Read the model definition and answer for the solid it produces. Units are mm, in the model's axes. Face numbers are marked on the shaded views. A direction names the side the tool comes from. Coordinates: 2 decimals unless noted, no trailing zeros. Order: outer loops, then holes, each group sorted by start corner. A loop starts at its lowest first (then second) coordinate and runs counter-clockwise, first axis right, second up. Notation, with made-up numbers: (-28.5, 16) -> (-15.5, 16) arc R34 cw to (-15.5, 49) -> close; hole circle Ø4 at (83.25, 79). An arc over 180 degrees is marked (long way). Use CSV: the item, a comma, the result in double quotes.
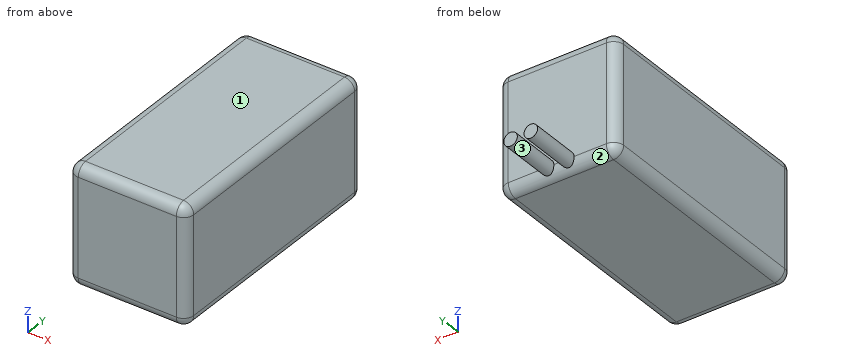
Autodesk Inventor part; units mm, degrees
ref_plane "YZ Plane" through (0, 0, 0) normal (1, 0, 0) x (0, 1, 0)
ref_plane "XZ Plane" through (0, 0, 0) normal (0, 1, 0) x (-1, 0, 0)
ref_plane "XY Plane" through (0, 0, 0) normal (0, 0, 1) x (1, 0, 0)
sketch "Sketch1" plane through (0, 0, 0) normal (0, 1, 0) x (-1, 0, 0)
  line L0 (17.5, 17.5) -> (-17.5, 17.5)
  line L1 (-17.5, 17.5) -> (-17.5, -17.5)
  line L2 (-17.5, -17.5) -> (17.5, -17.5)
  line L3 (17.5, -17.5) -> (17.5, 17.5)
  line L4 (17.5, 17.5) -> (-17.5, -17.5) construction
  line L5 (-17.5, 17.5) -> (17.5, -17.5) construction
  line L6 (0, -17.5) -> (0, -14.5) construction
  line L7 (0, -14.5) -> (3, -14.5) construction
  circle A0 centre (3, -14.5) radius 2
  circle A1 centre (-3, -14.5) radius 2
  point P0 (0, 0)
  dimension "d0" = 35
  dimension "d1" = 35
  dimension "d5" = 3
  dimension "d6" = 3
  dimension "d7" = 4
extrude "Extrusion1" add sketch "Sketch1" along normal blind 72 contours L3 L2 L1 L0 | A0 | A1
extrude "Extrusion2" add sketch "Sketch1" along normal blind 15 from surface at 72 contours A0 | A1
fillet "Fillet1" radius 3 12 edges at (17.5, 36, 17.5) (17.5, 36, -17.5) (-17.5, 36, 17.5) (-17.5, 36, -17.5) (17.5, 72, 0) (0, 72, 17.5) (0, 72, -17.5) (-17.5, 72, 0) (17.5, 0, 0) (0, 0, 17.5) (-17.5, 0, 0) (0, 0, -17.5)
properties part number "Tattu 14,8V 1550 mAh 100C LiPo-Akku XT60"
Item 1: A tool of negligible diameter and unlimited length cuts with its end or side. For the marked faces 1, 2 and 3, from which of +Z, -Z, +X, -X, +Y, -Y can it reach the whole face along a straight path? Write none if from no direction.
Return value:
face 1,"+Z, +X, -X, +Y, -Y"
face 2,"-Z, +Y"
face 3,"+Y"
Item 2: This flat-tipped pin is pushed along its axis until it touches: P1, Ø1.5, axis at x = 0, z = -2.5, coming from the +Y side. Where does it stop, or does it pass through?
Return value:
P1,"stops at y = 72"
Item 3: Straight lines are drawn through the part: line 1 along Y through (x, z) = (-2.5, -11); line 2 along X through (y, z) = (21.5, 16); line 3 along Y through (x, z) = (-1, 16). For each, find the intervals that lie inside material, in ascending order.
Return value:
line 1,"y = 0 to 72"
line 2,"x = -17.1 to 17.1"
line 3,"y = 0.4 to 71.6"
Item 4: Find section B-B, the plane z = 8. Give the vertices of the cut face in (x, y).
Return value:
outline,"(-17.5, 3) arc R3 ccw to (-14.5, 0) -> (14.5, 0) arc R3 ccw to (17.5, 3) -> (17.5, 69) arc R3 ccw to (14.5, 72) -> (-14.5, 72) arc R3 ccw to (-17.5, 69) -> close"
Item 5: Find section C-C, the plane x = -3. Give the vertices of the cut face in (y, z), then the cut area to 3 significant figures.
Return value:
outline,"(0, -14.5) arc R3 ccw to (3, -17.5) -> (69, -17.5) arc R3 ccw to (71.24, -16.5) -> (87, -16.5) -> (87, -12.5) -> (72, -12.5) -> (72, 14.5) arc R3 ccw to (69, 17.5) -> (3, 17.5) arc R3 ccw to (0, 14.5) -> close"
area,"2,570 mm^2"
Item 6: Find section A-A, the plane x = -13. Give the vertices of the cut face in (y, z), then the cut area to 3 significant figures.
Return value:
outline,"(0, -14.5) arc R3 ccw to (3, -17.5) -> (69, -17.5) arc R3 ccw to (72, -14.5) -> (72, 14.5) arc R3 ccw to (69, 17.5) -> (3, 17.5) arc R3 ccw to (0, 14.5) -> close"
area,"2,510 mm^2"
